Autodesk Inventor part; units mm, degrees
ref_plane "YZ Plane" through (0, 0, 0) normal (1, 0, 0) x (0, 1, 0)
ref_plane "XZ Plane" through (0, 0, 0) normal (0, 1, 0) x (-1, 0, 0)
ref_plane "XY Plane" through (0, 0, 0) normal (0, 0, 1) x (1, 0, 0)
sketch "Sketch1" plane through (0, 0, 0) normal (0, 1, 0) x (-1, 0, 0)
  circle A0 centre (0, 0) radius 190.5
  dimension "d0" = 381
extrude "Extrusion1" add sketch "Sketch1" along normal blind 25.4
sketch "Sketch2" plane through (0, 25.4, 0) normal (0, 1, 0) x (1, 0, 0)
  circle A0 centre (0, 0) radius 76.2
  dimension "d3" = 152.4
extrude "Extrusion2" add sketch "Sketch2" along normal blind 50.8
sketch "Sketch3" plane through (0, 0, 0) normal (0, 1, 0) x (-1, 0, 0)
  circle A0 centre (0, 0) radius 66.04
  dimension "d6" = 132.08
extrude "Extrusion3" cut sketch "Sketch3" along normal up to next
sketch "Sketch10" plane through (0, 0, 0) normal (0, 0, 1) x (1, 0, 0)
  line L0 (25.4, 12.7) -> (-25.4, 12.7)
  circle A0 centre (127, 12.7) radius 6.35
  circle A1 centre (-127, 12.7) radius 6.35
  point P0 (0, 0)
  dimension "d37" = 12.7
  dimension "d38" = 12.7
  dimension "d41" = 254
extrude "Extrusion10" cut sketch "Sketch10" along normal mid plane 508
properties part number "Top1"
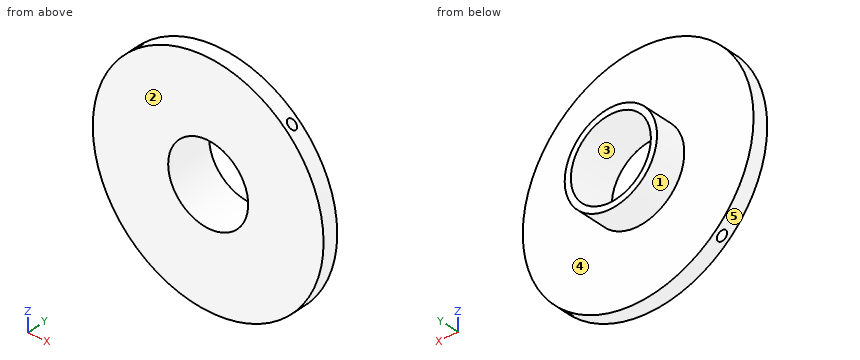
Input: part model. Units: mm. Frame: model coordinates. Face numbers are marked on the shaded views. A direction names the side the tool comes from. Give positions to 0.01 mm unless a question says otherwise; leave off trailing zeros. Order: outer loops, then holes, each group sorted by start corner. A loop starts at its lowest first (then second) coordinate and runs counter-clockwise, first axis right, second up. Notation, with made-up numbers: (79.5, 51.25) - (119.5, 51.25) arc R15 cw to (119.5, 71.25) - close; hole circle Ø3 at (25, 1.25). An arc over 180 degrees is marked (long way). Put each result on its own line as item: value.
Item 1: Section query A-A, the plane x = 0. Return loops of the section in (y, z), then the cut area to 3 significant figures.
Found:
outline: (0, -190.5) - (25.4, -190.5) - (25.4, -76.2) - (76.2, -76.2) - (76.2, -66.04) - (0, -66.04) - close; (0, 66.04) - (76.2, 66.04) - (76.2, 76.2) - (25.4, 76.2) - (25.4, 190.5) - (0, 190.5) - close
area: 7,350 mm^2
Item 2: Section query D-D, the plane x = -127. Return loops of the section in (y, z), then the cut area to 3 significant figures.
Found:
outline: (0, -141.99) - (6.35, -141.99) - (6.35, 141.99) - (0, 141.99) - close; (19.05, -141.99) - (25.4, -141.99) - (25.4, 141.99) - (19.05, 141.99) - close
area: 3,610 mm^2
Item 3: Draft query along Z for the marked faces 1, 2 and 3. Return one class per face: +Z half, -Z half, draft (parallel to the pull), parting line (faces both ways), or undercut.
Found:
face 1: parting line
face 2: draft
face 3: undercut
Item 4: Section query B-B, the plane z = 71. Return loops of the section in (x, y), then the cut area to 3 significant figures.
Found:
outline: (-176.77, 0) - (176.77, 0) - (176.77, 25.4) - (27.67, 25.4) - (27.67, 76.2) - (-27.67, 76.2) - (-27.67, 25.4) - (-176.77, 25.4) - close; hole circle Ø12.7 at (-127, 12.7); hole circle Ø12.7 at (127, 12.7)
area: 11,500 mm^2
Item 5: Section query C-C, the plane y = 30.5. Return loops of the section in (x, z).
Found:
outline: circle Ø152.4 at (0, 0); hole circle Ø132.08 at (0, 0)
Item 6: Contact query for flat-ended pins moving along their axis: pin 1 (5 mm diameter, centred on y = 24.5, z = -71.5, fed in from +X); pin 2 (1.5 mm diameter, centred on x = 11, y = 48.5, fed in from +Z); pin 3 (5 mm diameter, centred on y = 28.5, z = -82, fed in from -X); pin 4 (8 mm diameter, centred on x = 116.5, z = 12.5, fed in from +Y). Output: stop coordinate, or through.
Found:
pin 1: stops at x = 177.56
pin 2: stops at z = 75.51
pin 3: passes through
pin 4: stops at y = 25.4
Item 7: Access query for the marked faces 4 and 5. Directions: +Z, -Z, +X, -X, +Y, -Y. A direction counts if a zero-diameter tool reaches every point of the face in a straight line with its end or side. Return the directions, or none.
Found:
face 4: +Y
face 5: +Y, -Y
Item 8: Ray query, L1, parallel to Y at x = 127, z = -38.5; L2, parallel to Z at x = 0, y = 16; L3, parallel to X at y = 7, z = 29. Return the intervals inside material, ascending. Write a range as from..to.
Found:
L1: y = 0..6.35, 19.05..25.4
L2: z = -190.5..-66.04, 66.04..190.5
L3: x = -188.28..-129.8, -124.2..-59.33, 59.33..124.2, 129.8..188.28
